```python
from build123d import *

# Parameters (mm, degrees)
SKETCH1_W           = 6.8
SKETCH1_H           = 2.2
BOSS_EXTRUDE1_DEPTH = 8
CUT_EXTRUDE1_DEPTH  = 8
FILLET1_R           = 0.15


with BuildPart() as part:
    # Sketch1 → Boss-Extrude1 (new body)
    with BuildSketch(Plane.XY):
        Rectangle(SKETCH1_W, SKETCH1_H)
    extrude(amount=BOSS_EXTRUDE1_DEPTH)

    # Sketch2 → Cut-Extrude1 (cut)
    with BuildSketch(Plane(origin=(0, 1.1, 0), x_dir=(1, 0, 0), z_dir=(0, 1, 0))):
        with BuildLine():
            Line((-3.4, -7.5), (-4.338442441, -8.7499714))
            Line((-4.338442441, -8.7499714), (5.303990533, -8.971786502))
            Line((5.303990533, -8.971786502), (3.4, -7.5))
            ThreePointArc((3.4, -7.5), (0, -7.952490287), (-3.4, -7.5))
        make_face()
    extrude(amount=-CUT_EXTRUDE1_DEPTH, mode=Mode.SUBTRACT)

    # Fillet1
    fillet1_edges = [part.edges().sort_by_distance(p)[0] for p in [
        (-3.4, 1.1, 3.75),
        (3.4, 1.1, 3.75),
        (3.4, -1.1, 3.75),
        (-3.4, -1.1, 3.75),
        (0, -1.1, 7.952490287),
        (-3.4, 0, 7.5),
        (0, 1.1, 7.952490287),
        (3.4, 0, 7.5),
        (0, 1.1, 0),
        (3.4, 0, 0),
        (0, -1.1, 0),
        (-3.4, 0, 0),
    ]]
    fillet(fillet1_edges, radius=FILLET1_R)


solid = part.part
```
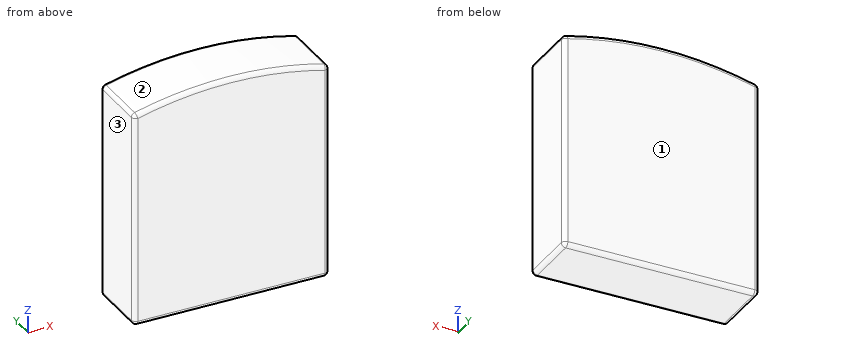
Can you work these out from the model? Positions are in its coordinate system, mm. Face numbers are marked on the shaded views. Round coordinates to 2 decimals unless told otherwise and drop trailing zeros. Order: outer loops, then holes, each group sorted by start corner. A loop starts at its lowest first (then second) coordinate and runs counter-clockwise, first axis right, second up.
(1) If I drill on L1, parallel to Z at x = 0.5, y = 0.7; L2, parallel to Z at x = 2.5, y = 0.8, over which ranges is the centre line in solid material (lowest first)?
Results are:
L1: z = 0 to 7.94
L2: z = 0 to 7.71
(2) We'd pull the mould along X, two halves only. Please class the marked faces 1, 2 and 3: +X half, -X half, draft (parallel to the pull), parting line (faces both ways), or undercut.
Results are:
face 1: draft
face 2: parting line
face 3: -X half
(3) If we section it at A-A (y = -0.4): Please give me the cut outline in (x, z).
Results are:
outline: (-3.4, 0.15) arc R0.15 ccw to (-3.25, 0) - (3.25, 0) arc R0.15 ccw to (3.4, 0.15) - (3.4, 7.38) arc R0.15 ccw to (3.29, 7.53) arc R13 ccw to (-3.29, 7.53) arc R0.15 ccw to (-3.4, 7.38) - close
